Autodesk Inventor part; units mm, degrees
ref_plane "YZ Plane" through (0, 0, 0) normal (1, 0, 0) x (0, 1, 0)
ref_plane "XZ Plane" through (0, 0, 0) normal (0, 1, 0) x (-1, 0, 0)
ref_plane "XY Plane" through (0, 0, 0) normal (0, 0, 1) x (1, 0, 0)
sketch "Sketch1" plane through (0, 0, 0) normal (1, 0, 0) x (0, 1, 0)
  line L0 (3.6662, 6.35) -> (7.3323, 0)
  line L1 (7.3323, 0) -> (3.6662, -6.35)
  line L2 (3.6662, -6.35) -> (-3.6662, -6.35)
  line L3 (-3.6662, -6.35) -> (-7.3323, 0)
  line L4 (-7.3323, 0) -> (-3.6662, 6.35)
  line L5 (-3.6662, 6.35) -> (3.6662, 6.35)
  point P0 (0, 0)
  point P1 (0, 0)
  dimension "d0" = 12.7
extrude "Extrusion1" add sketch "Sketch1" along normal mid plane 80.3402
sketch "Sketch2" plane through (40.1701, 0, 0) normal (1, 0, 0) x (0, 0, -1)
  line L0 (-6.35, -3.6662) -> (0, -7.3323)
  line L1 (0, -7.3323) -> (6.35, -3.6662)
  line L2 (6.35, -3.6662) -> (6.35, 3.6662)
  line L3 (6.35, 3.6662) -> (0, 7.3323)
  line L4 (0, 7.3323) -> (-6.35, 3.6662)
  line L5 (-6.35, 3.6662) -> (-6.35, -3.6662)
  circle A0 centre (0, 0) radius 6.35
  point P0 (-3.175, 5.4993)
  point P1 (3.175, 5.4993)
  point P2 (6.35, 0)
  point P3 (3.175, -5.4993)
  point P4 (-3.175, -5.4993)
  point P5 (-6.35, 0)
  dimension "d3" = 12.7
extrude "Extrusion2" cut sketch "Sketch2" against normal blind 7.9375 contours L5 A0 L0 | A0 L1 L0 | L5 L4 A0 | A0 L2 L1 | L4 L3 A0 | A0 L3 L2
sketch "Sketch4" plane through (-40.1701, 0, 0) normal (-1, 0, 0) x (0, 0, 1)
  point P0 (0, 0)
  point P1 (0, 0)
hole "Hole1" at (-40.1701, 0, 0) direction (1, 0, 0) diameter 3.9624 depth 13.6144 tip angle 118
properties part number "EL2-CGB-004" material "Aluminum 6061"
Could you check a few things on this model? Use its own coordinates, in mm. A direction names the side the tool comes from. Round coordinates to 2 decimals unless told otherwise and drop trailing zeros. Loops run counter-clockwise (first coordinate to the right, second up) from the corner with the lowest first, then second, coordinate; pieces in that order, holes last. Notation, with made-up numbers: (-23, -30.5) -> (9, -30.5) arc R20 cw to (9, -21.5) -> close; hole circle Ø8 at (52, -3.75). An arc over 180 degrees is marked (long way). Use CSV: the item, a comma, the result in double quotes.
(1) For faces 4 (the flat face through (32.233, -7, 0)), 5 (the flat face through (32.233, -3, -6)), 6 (the flat face through (32.233, 3, -6)), 7 (the flat face through (32.233, 3, 6)), which set-ups out of +Z, -Z, +X, -X, +Y, -Y let a thin tool reach every point of the face, with its end or its side?
Return value:
face 4,"+X, -Y"
face 5,"-Z, +X, -Y"
face 6,"-Z, +X, +Y"
face 7,"+Z, +X, +Y"
(2) Suppose I cut it at A-A on x = 9.5. Write out the boundary of the cut face in (y, z), plus the area to 3 significant figures.
Return value:
outline,"(-7.33, 0) -> (-3.67, -6.35) -> (3.67, -6.35) -> (7.33, 0) -> (3.67, 6.35) -> (-3.67, 6.35) -> close"
area,"140 mm²"
(3) Suppose I cut it at B-B on y = -4.75. Write out the boundary of the cut face in (x, z).
Return value:
outline,"(-40.17, -4.47) -> (32.23, -4.47) -> (32.23, -4.21) -> (40.17, -4.21) -> (40.17, 4.21) -> (32.23, 4.21) -> (32.23, 4.47) -> (-40.17, 4.47) -> close"
(4) Will these pins go through, and if not, where does the flat tip stop? pin 1 Ø3.5 at (y, z) = (0, 0) entering from -X; pin 2 Ø0.5 at (y, z) = (-7, 0.5) entering from +X; pin 3 Ø5 at (x, z) = (-17.5, -4.5) entering from -Y.
Return value:
pin 1,"stops at x = -26.42"
pin 2,"stops at x = 32.23"
pin 3,"stops at y = -6.18"
(5) If I drill on probe 1 along Y at (x, z) = (-32.5, 0); probe 2 along Z at (x, y) = (-34.5, 0); probe 3 along Z at (x, y) = (22, -5.5), over which ranges is the centre line in solid material (lowest first)? Write a range as [from, to].
Return value:
probe 1,"y = [-7.33, -1.98], [1.98, 7.33]"
probe 2,"z = [-6.35, -1.98], [1.98, 6.35]"
probe 3,"z = [-3.17, 3.17]"
(6) If we mould it in two halves opening along Z, with no side actions, what happens to faces 1 (the cylindrical face through (36.26, -6.2, 1.38)), 2 (the flat face through (32.233, -3, 6)), 3 (the conical face through (-25.572, -0.336, -0.075))? For each: +Z half, -Z half, draft (parallel to the pull), parting line (faces both ways), or undercut.
Return value:
face 1,"parting line"
face 2,"draft"
face 3,"undercut"
(7) Suppose I cut it at C-C on x = 35. Write out the boundary of the cut face in (y, z), plus the area to 3 significant figures.
Return value:
outline,"circle Ø12.7 at (0, 0)"
area,"127 mm²"
